```python
from build123d import *

# Parameters (mm, degrees)
SKETCH1_W               = 807.72
SKETCH1_H               = 401.32
BOSS_EXTRUDE1_DEPTH     = 25.4
SKETCH1_3_W             = 807.72
SKETCH1_3_H             = 401.32
BOSS_EXTRUDE2_DEPTH     = 243.84
SKETCH2_R               = 60.96
BOSS_EXTRUDE3_DEPTH     = 45.72
SKETCH3_R               = 82.55
SKETCH3_R_2             = 52.07
BOSS_EXTRUDE4_DEPTH     = 243.84
BOSS_EXTRUDE5_DEPTH     = 167.64
CUT_EXTRUDE3_DEPTH      = 25.4
CUT_EXTRUDE3_DEPTH_BACK = 25.4
SKETCH2_6_R             = 30.48


with BuildPart() as part:
    # Sketch1 → Boss-Extrude1 (new body)
    # profile 1 of 2: a face of its own
    with BuildSketch(Plane(origin=(0, 0, 0), x_dir=(1, 0, 0), z_dir=(0, 1, 0))):
        with Locations((-96.713172489, -45.20036793)):
            Rectangle(SKETCH1_W, SKETCH1_H)
        Polygon((271.586827511, 41.15963207), (276.666827511, 41.15963207), (276.666827511, -131.56036793), (271.586827511, -131.56036793), (271.586827511, -162.04036793), (276.666827511, -162.04036793), (276.666827511, -215.38036793), (-470.093172489, -215.38036793), (-470.093172489, -162.04036793), (-465.013172489, -162.04036793), (-465.013172489, -131.56036793), (-470.093172489, -131.56036793), (-470.093172489, 41.15963207), (-465.013172489, 41.15963207), (-465.013172489, 71.63963207), (-470.093172489, 71.63963207), (-470.093172489, 124.97963207), (-416.753172489, 124.97963207), (-416.753172489, 119.89963207), (-386.273172489, 119.89963207), (-386.273172489, 124.97963207), (-206.418642564, 124.97963207), (-206.418642564, 119.89963207), (-175.951162142, 119.89963207), (-175.951162142, 124.97963207), (-17.475182836, 124.97963207), (-17.475182836, 119.89963207), (12.992297586, 119.89963207), (12.992297586, 124.97963207), (192.846827511, 124.97963207), (192.846827511, 119.89963207), (223.326827511, 119.89963207), (223.326827511, 124.97963207), (276.666827511, 124.97963207), (276.666827511, 71.63963207), (271.586827511, 71.63963207), align=None, mode=Mode.SUBTRACT)
    # profile 2 of 2: a face of its own
    with BuildSketch(Plane(origin=(0, 0, 0), x_dir=(1, 0, 0), z_dir=(0, 1, 0))):
        Polygon((276.666827511, 41.15963207), (276.666827511, -131.56036793), (271.586827511, -131.56036793), (271.586827511, -162.04036793), (276.666827511, -162.04036793), (276.666827511, -215.38036793), (-470.093172489, -215.38036793), (-470.093172489, -162.04036793), (-465.013172489, -162.04036793), (-465.013172489, -131.56036793), (-470.093172489, -131.56036793), (-470.093172489, 41.15963207), (-465.013172489, 41.15963207), (-465.013172489, 71.63963207), (-470.093172489, 71.63963207), (-470.093172489, 124.97963207), (-416.753172489, 124.97963207), (-416.753172489, 119.89963207), (-386.273172489, 119.89963207), (-386.273172489, 124.97963207), (-206.418642564, 124.97963207), (-206.418642564, 119.89963207), (-175.951162142, 119.89963207), (-175.951162142, 124.97963207), (-17.475182836, 124.97963207), (-17.475182836, 119.89963207), (12.992297586, 119.89963207), (12.992297586, 124.97963207), (192.846827511, 124.97963207), (192.846827511, 119.89963207), (223.326827511, 119.89963207), (223.326827511, 124.97963207), (276.666827511, 124.97963207), (276.666827511, 71.63963207), (271.586827511, 71.63963207), (271.586827511, 41.15963207), align=None)
    extrude(amount=BOSS_EXTRUDE1_DEPTH)

    # Sketch1<3> → Boss-Extrude2 (add)
    with BuildSketch(Plane(origin=(0, 0, 0), x_dir=(1, 0, 0), z_dir=(0, 1, 0))):
        with Locations((-96.713172489, -45.20036793)):
            Rectangle(SKETCH1_3_W, SKETCH1_3_H)
        Polygon((-416.753172489, 124.97963207), (-416.753172489, 119.89963207), (-386.273172489, 119.89963207), (-386.273172489, 124.97963207), (-206.418642564, 124.97963207), (-206.418642564, 119.89963207), (-175.951162142, 119.89963207), (-175.951162142, 124.97963207), (-17.475182836, 124.97963207), (-17.475182836, 119.89963207), (12.992297586, 119.89963207), (12.992297586, 124.97963207), (192.846827511, 124.97963207), (192.846827511, 119.89963207), (223.326827511, 119.89963207), (223.326827511, 124.97963207), (276.666827511, 124.97963207), (276.666827511, 71.63963207), (271.586827511, 71.63963207), (271.586827511, 41.15963207), (276.666827511, 41.15963207), (276.666827511, -131.56036793), (271.586827511, -131.56036793), (271.586827511, -162.04036793), (276.666827511, -162.04036793), (276.666827511, -215.38036793), (-470.093172489, -215.38036793), (-470.093172489, -162.04036793), (-465.013172489, -162.04036793), (-465.013172489, -131.56036793), (-470.093172489, -131.56036793), (-470.093172489, 41.15963207), (-465.013172489, 41.15963207), (-465.013172489, 71.63963207), (-470.093172489, 71.63963207), (-470.093172489, 124.97963207), align=None, mode=Mode.SUBTRACT)
    extrude(amount=-BOSS_EXTRUDE2_DEPTH)

    # Sketch2 → Boss-Extrude3 (add)
    with BuildSketch(Plane(origin=(0, 25.4, 0), x_dir=(1, 0, 0), z_dir=(0, 1, 0))):
        with Locations(Location((-401.513172489, 56.39963207, 0), (0, 0, 270))):
            Circle(SKETCH2_R)
        with Locations(Location((-198.313172489, 56.39963207, 0), (0, 0, 270))):
            Circle(SKETCH2_R)
        with Locations(Location((-198.313172489, -146.80036793, 0), (0, 0, 270))):
            Circle(SKETCH2_R)
        with Locations(Location((-401.513172489, -146.80036793, 0), (0, 0, 270))):
            Circle(SKETCH2_R)
        with Locations(Location((208.086827511, -146.80036793, 0), (0, 0, 270))):
            Circle(SKETCH2_R)
        with Locations(Location((4.886827511, -146.80036793, 0), (0, 0, 270))):
            Circle(SKETCH2_R)
        with Locations(Location((4.886827511, 56.39963207, 0), (0, 0, 270))):
            Circle(SKETCH2_R)
        with Locations(Location((208.086827511, 56.39963207, 0), (0, 0, 270))):
            Circle(SKETCH2_R)
    extrude(amount=BOSS_EXTRUDE3_DEPTH)

    # Sketch3 → Boss-Extrude4 (add)
    # profile 1 of 3: a face of its own
    with BuildSketch(Plane.XZ):
        with Locations(Location((106.486827511, 45.20036793, 0), (0, 0, 90))):
            Circle(SKETCH3_R)
        with Locations(Location((106.486827511, 45.20036793, 0), (0, 0, 90))):
            Circle(SKETCH3_R_2, mode=Mode.SUBTRACT)
    # profile 2 of 3: a face of its own
    with BuildSketch(Plane.XZ):
        with Locations(Location((-96.713172489, 45.20036793, 0), (0, 0, 90))):
            Circle(SKETCH3_R)
        with Locations(Location((-96.713172489, 45.20036793, 0), (0, 0, 90))):
            Circle(SKETCH3_R_2, mode=Mode.SUBTRACT)
    # profile 3 of 3: a face of its own
    with BuildSketch(Plane.XZ):
        with Locations(Location((-299.913172489, 45.20036793, 0), (0, 0, 90))):
            Circle(SKETCH3_R)
        with Locations(Location((-299.913172489, 45.20036793, 0), (0, 0, 90))):
            Circle(SKETCH3_R_2, mode=Mode.SUBTRACT)
    extrude(amount=BOSS_EXTRUDE4_DEPTH)

    # Sketch3<4> → Boss-Extrude5 (add)
    with BuildSketch(Plane.XZ):
        with BuildLine():
            Line((-110.683172489, 215.38036793), (-110.683172489, 126.55970421))
            ThreePointArc((-110.683172489, 126.55970421), (-96.713172489, 127.75036793), (-82.743172489, 126.55970421))
            Line((-82.743172489, 126.55970421), (-82.743172489, 215.38036793))
            Line((-82.743172489, 215.38036793), (-110.683172489, 215.38036793))
        make_face()
        with BuildLine():
            ThreePointArc((-82.743172489, -36.158968351), (-96.713172489, -37.34963207), (-110.683172489, -36.158968351))
            Line((-110.683172489, -36.158968351), (-110.683172489, -124.97963207))
            Line((-110.683172489, -124.97963207), (-82.743172489, -124.97963207))
            Line((-82.743172489, -124.97963207), (-82.743172489, -36.158968351))
        make_face()
    extrude(amount=BOSS_EXTRUDE5_DEPTH)

    # Sketch2<6> → Cut-Extrude3 (cut, two sides: drawn at the far end of the back side and taken through both)
    with BuildSketch(Plane(origin=(0, 25.4, 0), x_dir=(1, 0, 0), z_dir=(0, 1, 0)).offset(-CUT_EXTRUDE3_DEPTH_BACK)):
        with Locations(Location((-401.513172489, 56.39963207, 0), (0, 0, 270))):
            Circle(SKETCH2_6_R)
        with Locations(Location((-198.313172489, 56.39963207, 0), (0, 0, 270))):
            Circle(SKETCH2_6_R)
        with Locations(Location((-198.313172489, -146.80036793, 0), (0, 0, 270))):
            Circle(SKETCH2_6_R)
        with Locations(Location((208.086827511, -146.80036793, 0), (0, 0, 270))):
            Circle(SKETCH2_6_R)
        with Locations(Location((208.086827511, 56.39963207, 0), (0, 0, 270))):
            Circle(SKETCH2_6_R)
        with Locations(Location((-401.513172489, -146.80036793, 0), (0, 0, 90))):
            Circle(SKETCH2_6_R)
        with Locations(Location((4.886827511, -146.80036793, 0), (0, 0, 270))):
            Circle(SKETCH2_6_R)
    extrude(amount=CUT_EXTRUDE3_DEPTH + CUT_EXTRUDE3_DEPTH_BACK, mode=Mode.SUBTRACT)


solid = part.part
```
The listing builds one solid part. Answer for the finished solid, in the listing's coordinates (mm). A direction names the side the tool comes from. Coordinates: 2 decimals unless noted, no trailing zeros. Loops run counter-clockwise (first coordinate to the right, second up) from the corner with the lowest first, then second, coordinate; pieces in that order, holes last. Notation, with made-up numbers: M -20,38.5 L 15,38.5 A10 ccw 15,55.5 Z; hole C -17,66.5 d9. An arc over 180 degrees is marked long. Answer as CSV lines item,"result". Start each with the question number.
(1) The part is cut by section C-C (z = 195.5). Give the vertices of the cut face in (x, y), and give its area (3 significant figures).
(2) The part is cut by section B-B (y = -21). State how many separate pieces and enclosed holes the cut face has, and give its area (3 significant figures).
(3) The mould has two halves that part along Z. Classify faces 3 (the flat face through (-197, 71.12, 146)), 4 (the flat face through (102, -120, -124.98)): pulls with the +Z half, pulls with the -Z half, needs draft (parallel to the pull), parting line crosses it, or undercut.
(4) The part is cut by section A-A (x = -119). Give the vertices of the cut face in (y, z), and give its area (3 significant figures).
(5) Given pin 1 (3 mm diameter, centred on y = 28, z = 165.5, fed in from +X); pin 2 (10 mm diameter, centred on x = -278.5, z = 131.5, fed in from +Y), each flat-ended and moving along its own axis, determine where each tip first touches the part or whether it passes through.
(6) Find the intervals of material crossed by L1, parallel to X at y = -10.5, z = 144; L2, parallel to X at y = -77.5, z = -110.5; L3, parallel to Z at x = 10, y = -188, in increasing order. Write a range as [from, to].
(7) For faces 1 (the flat face through (307.147, -107, 48)), 2 (the cylindrical face through (-65.096, -120.213, 121.456)), determine the directions among +Z, -Z, +X, -X, +Y, -Y from which every point of the face is accessible in a straight line to the end or side of a thin tool.
Determined:
1,outline,"M -500.57,-243.84 L -470.09,-243.84 L -470.09,0 L -110.68,0 L -110.68,-167.64 L -82.74,-167.64 L -82.74,0 L 276.67,0 L 276.67,-243.84 L 307.15,-243.84 L 307.15,25.4 L 244.75,25.4 L 244.75,71.12 L 171.42,71.12 L 171.42,25.4 L 41.55,25.4 L 41.55,71.12 L -31.78,71.12 L -31.78,25.4 L -161.65,25.4 L -161.65,71.12 L -234.98,71.12 L -234.98,25.4 L -364.85,25.4 L -364.85,71.12 L -438.18,71.12 L -438.18,25.4 L -500.57,25.4 Z"
1,area,"53,500 mm2"
2,separate pieces,"3"
2,enclosed holes,"5"
2,area,"115,000 mm2"
3,face 3,"needs draft"
3,face 4,"undercut"
4,outline,"M -243.84,-155.46 L 25.4,-155.46 L 25.4,245.86 L -243.84,245.86 L -243.84,215.38 L 0,215.38 L 0,124.68 L -243.84,124.68 L -243.84,92.26 L 0,92.26 L 0,-1.86 L -243.84,-1.86 L -243.84,-34.28 L 0,-34.28 L 0,-124.98 L -243.84,-124.98 Z"
4,area,"40,900 mm2"
5,pin 1,"x = 266.57"
5,pin 2,"y = 25.4"
6,L1,"[-500.57, -465.01], [-110.68, -82.74], [271.59, 307.15]"
6,L2,"[-500.57, -470.09], [-110.68, -82.74], [276.67, 307.15]"
6,L3,"[-155.46, -119.9], [215.38, 245.86]"
7,face 1,"+Z, -Z, +X, +Y, -Y"
7,face 2,"-Y"
